from build123d import *

# Parameters (mm, degrees)
F1_DEPTH = 38.1
F2_W     = 19.05
F2_H     = 9.525
F3_DEPTH = 19.05


with BuildPart() as f1:
    # F0 (on Right) → F1 (new body)
    with BuildSketch(Plane.YZ):
        Polygon((152.4, -6.35), (114.3, 19.05), (-114.3, 19.05), (-152.4, -6.35), (-152.4, -19.05), (-101.6, -19.05), (76.2, -19.05), (152.4, -19.05), align=None)
    extrude(amount=F1_DEPTH)

    # F2 (on face) → F3 (cut)
    with BuildSketch(Plane.XY.offset(19.05)):
        with Locations((19.05, 4.7625)):
            Rectangle(F2_W, F2_H)
        with Locations((19.05, -4.7625)):
            Rectangle(F2_W, F2_H)
    extrude(amount=-F3_DEPTH, mode=Mode.SUBTRACT)


with BuildPart() as f4_1:
    # F4: copy of F1
    add(f1.part)


solid = f1.part
Design review of the part built by this model. Coordinates are the model's own, in mm. A direction names the side the tool comes from. Give positions to 0.01 mm unless a question says otherwise; leave off trailing zeros. Loops run counter-clockwise (first coordinate to the right, second up) from the corner with the lowest first, then second, coordinate; pieces in that order, holes last. Notation, with made-up numbers: M 86.5,81 L 112.5,81 A9 cw 112.5,92 Z; hole C -22,-19.5 d6. An arc over 180 degrees is marked long. Answer as a JSON object with one key per item and string values.
Item 1: We need section D-D (x = 4.5). State the section outline as (y, z) points.
Output values:
{"outline": "M -152.4,-19.05 L 152.4,-19.05 L 152.4,-6.35 L 114.3,19.05 L -114.3,19.05 L -152.4,-6.35 Z"}
Item 2: Mouldability with a two-part tool opening along Y and no side actions: class faces 1 (the face through (19, 152.4, -13)), 2 (the face through (19, -152.4, -13)), 3 (the face through (0, -2, 0)), 4 (the face through (9.525, 0, 10)) as pulls with the +Y half, pulls with the -Y half, needs draft (parallel to the pull), parting line crosses it, or undercut.
Output values:
{"face 1": "pulls with the +Y half", "face 2": "pulls with the -Y half", "face 3": "needs draft", "face 4": "undercut"}
Item 3: We need section A-A (x = 25). State the section outline as (y, z) points (3 decimals).
Output values:
{"outline": "M -152.4,-19.05 L 152.4,-19.05 L 152.4,-6.35 L 114.3,19.05 L 9.525,19.05 L 9.525,0 L -9.525,0 L -9.525,19.05 L -114.3,19.05 L -152.4,-6.35 Z"}
Item 4: Machinability: for faces 5 (the face through (19, -9.525, 10)), 6 (the face through (18.78, -133.08, 6.53)), which of the approach directions +Z, -Z, +X, -X, +Y, -Y give a long, thin tool a straight path to every point of the face, cutting with its end or side? Answer none if there is none.
Output values:
{"face 5": "+Z", "face 6": "+Z, +X, -X, -Y"}
Item 5: Wall thickness on line 1 along X through (y, z) = (-4, 12.5) (3 decimals); line 2 along Y through (x, z) = (28, 16.5) (3 decimals); line 3 along Y through (x, z) = (31.5, -4) (3 decimals): over which ranges is each line inside the solid? List them lowest first.
Output values:
{"line 1": "x = 0 to 9.525, 28.575 to 38.1", "line 2": "y = -118.125 to -9.525, 9.525 to 118.125", "line 3": "y = -148.875 to 148.875"}
Item 6: We need section C-C (y = 130.5). State the section outline as (x, z) points.
Output values:
{"outline": "M 0,-19.05 L 38.1,-19.05 L 38.1,8.25 L 0,8.25 Z"}
Item 7: For P1, Ø5.5, axis at y = -4, z = 7, coming from the -X side; P2, Ø5.5, axis at x = 17.5, z = 6.5, coming from the -Y side; P3, Ø9.5, axis at x = 14.5, z = 10, coming from the +Y side; P4, Ø10, axis at x = 15, z = -0.5, coming from the +Y side (3 decimals), all flat-tipped, find the tip position at first contact; note any pin that passes through.
Output values:
{"P1": "stops at x = 0", "P2": "stops at y = -137.25", "P3": "stops at y = 135", "P4": "stops at y = 151.125"}
Item 8: We need section B-B (z = 9.5). State the section outline as (x, y) points (3 decimals).
Output values:
{"outline": "M 0,-128.625 L 38.1,-128.625 L 38.1,128.625 L 0,128.625 Z; hole M 9.525,-9.525 L 28.575,-9.525 L 28.575,9.525 L 9.525,9.525 Z"}
